from build123d import *

# Parameters (mm, degrees)
EXTRUDE_1_DEPTH           = 15
SKETCH_2_W                = 14
SKETCH_2_H                = 67.5
HOLE_WIZARD_1_D           = 85
HOLE_WIZARD_1_CBORE_D     = 111
HOLE_WIZARD_1_CBORE_DEPTH = 19
HOLE_WIZARD_2_D           = 3.242
HOLE_WIZARD_2_DEPTH       = 8
HOLE_WIZARD_2_TIP         = 0.973995063
CHAMFER_1_SIZE            = 0.999999999
CHAMFER_1_SIZE2           = 1.000000001
CHAMFER_2_SIZE            = 0.267949192
CHAMFER_2_SIZE2           = 1


with BuildPart() as part:
    # 草圖1 → 填料-伸長1 (new body)
    with BuildSketch(Plane(origin=(125, 0, 0), x_dir=(0, -1, 0), z_dir=(-1, 0, 0))):
        with BuildLine():
            Line((-41.158231255, -71.5), (41.158231255, -71.5))
            ThreePointArc((41.158231255, -71.5), (0, 82.5), (-41.158231255, -71.5))
        make_face()
    extrude(amount=-EXTRUDE_1_DEPTH)

    # 草圖2 → 旋轉1 (revolve)
    with BuildSketch(Plane.XY, mode=Mode.PRIVATE) as revolve_1_sk:
        with Locations((118, 33.75)):
            Rectangle(SKETCH_2_W, SKETCH_2_H)
    revolve(revolve_1_sk.sketch.rotate(Axis((111, 0, 0), (1, 0, 0)), 270), axis=Axis((111, 0, 0), (1, 0, 0)))

    # 鑽孔1 (through all)
    with Locations(Plane(origin=(140, 0, 0), x_dir=(0, 0, -1), z_dir=(1, 0, 0))):
        with Locations((0, 0)):
            CounterBoreHole(HOLE_WIZARD_1_D / 2, HOLE_WIZARD_1_CBORE_D / 2, HOLE_WIZARD_1_CBORE_DEPTH)

    # 鑽孔2
    with Locations(Plane(origin=(121, 0, 0), x_dir=(0, 0, -1), z_dir=(1, 0, 0))):
        with Locations((0, 50), (-50, 0), (0, -50), (50, 0)):
            Hole(HOLE_WIZARD_2_D / 2, depth=HOLE_WIZARD_2_DEPTH)
            with Locations((0, 0, -(HOLE_WIZARD_2_DEPTH + HOLE_WIZARD_2_TIP / 2))):  # 118° drill point
                Cone(0, HOLE_WIZARD_2_D / 2, HOLE_WIZARD_2_TIP, mode=Mode.SUBTRACT)

    # 導角1
    chamfer_1_edges = [part.edges().sort_by_distance(p)[0] for p in [
        (125, 0, 82.5),
        (140, 0, 82.5),
    ]]
    chamfer_1_side = [part.faces().sort_by_distance(p)[0] for p in [
        (132.5, 0, 82.5),
    ]]
    chamfer(chamfer_1_edges, length=CHAMFER_1_SIZE, length2=CHAMFER_1_SIZE2, reference=chamfer_1_side[0])

    # 導角2
    chamfer_2_edges = [part.edges().sort_by_distance(p)[0] for p in [
        (121, 0, -42.5),
    ]]
    chamfer_2_side = [part.faces().sort_by_distance(p)[0] for p in [
        (121, 0, 53.930222946),
    ]]
    chamfer(chamfer_2_edges, length=CHAMFER_2_SIZE, length2=CHAMFER_2_SIZE2, reference=chamfer_2_side[0])


solid = part.part
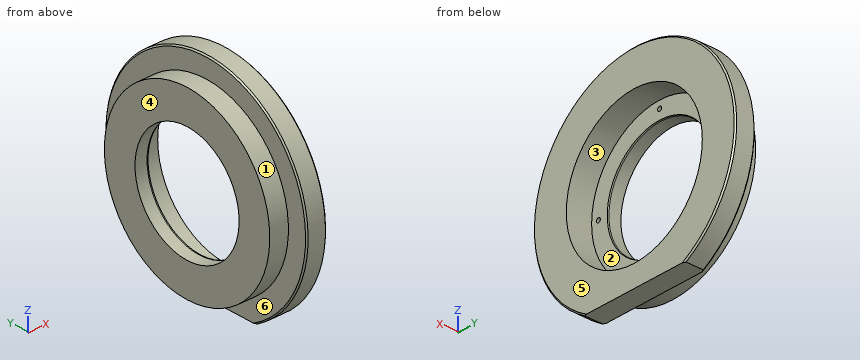
Part model, mm, in its own coordinate system. Face numbers are marked on the shaded views. A direction names the side the tool comes from. Give positions to 0.01 mm unless a question says otherwise; leave off trailing zeros. Loops run counter-clockwise (first coordinate to the right, second up) from the corner with the lowest first, then second, coordinate; pieces in that order, holes last. Notation, with made-up numbers: M 6,-36.75 L 35,-36.75 A17 cw 35,-12.75 Z; hole C 78,83 d7. An arc over 180 degrees is marked long. Put each result on its own line as item: value. Start each with the question number.
1) Saw through at B-B (x = 117). List the corners of the cut face in (y, z).
2) Probe probe 1 along Y at (x, z) = (116.5, 0); probe 2 along Z at (x, y) = (125.25, -43); probe 3 along Y at (x, z) = (129, 0). List the from-to ranges inside material, lowest first.
3) Pull direction Y, two halves, no side cores. Call the marked faces 1, 2, 3 and 4: +Y half, -Y half, draft (parallel to the pull), parting line (faces both ways), or undercut.
4) Flat gauge pins, fed straight in: pin 1 (3 mm diameter, centred on y = 1, z = 51, fed in from +X); pin 2 (2 mm diameter, centred on x = 132, z = -47.5, fed in from -Y); pin 3 (2 mm diameter, centred on y = -5, z = 41, fed in from -X); pin 4 (2.5 mm diameter, centred on y = -50, z = 0, fed in from +X). Where does each tip first touch, or does it go through?
5) 3-axis set-ups, long thin cutter, end or side, ignore diameter. For the marked faces 5 and 6: which of +Z, -Z, +X, -X, +Y, -Y reach the whole face in a straight line?
6) Saw through at A-A (x = 130.5). List the corners of the cut face in (y, z), then the cut area to 3 significant figures.
Numbers:
1. outline: C 0,0 d135; hole C -50,0 d3.24; hole C 0,0 d85; hole C 0,-50 d3.24; hole C 0,50 d3.24; hole C 50,0 d3.24
2. probe 1: -67.5 to -51.62, -48.38 to -42.5, 42.5 to 48.38, 51.62 to 67.5
2. probe 2: -69.53 to -35.09, 35.09 to 69.53
2. probe 3: -82.5 to -55.5, 55.5 to 82.5
3. face 1: parting line
3. face 2: undercut
3. face 3: undercut
3. face 4: draft
4. pin 1: x = 121
4. pin 2: y = -68.15
4. pin 3: through
4. pin 4: x = 112.78
5. face 5: +Z, -Z, +X, +Y, -Y
5. face 6: -X
6. outline: M -41.16,-71.5 L 41.16,-71.5 A82.5 ccw long Z; hole C 0,0 d111
6. area: 11,100 mm^2
